Read the model definition and answer for the solid it produces. Units are mm, in the model's axes. A direction names the side the tool comes from. Give positions to 0.01 mm unless a question says otherwise; leave off trailing zeros. Loops run counter-clockwise (first coordinate to the right, second up) from the corner with the lowest first, then second, coordinate; pieces in that order, holes last. Notation, with made-up numbers: (-32.5, -16) - (-28.5, -16) arc R23 ccw to (-28.5, 0) - close; hole circle Ø10 at (-9.5, 42). An arc over 180 degrees is marked (long way). Use a Markdown table: item, result. Add a question column.
Item 1: A cutting plane is placed at B-B (y = -6.5). Determine the outline of the cut face in (x, z).
Item 2: For a pull along Z with two mould halves and no side action, classify faces 4 (the face through (24.2, 0.1, 0)), 5 (the face through (4.5, 25, 22.2)), 6 (the face through (-9.52, 23.52, 21.88)) as +Z half, -Z half, draft (parallel to the pull), parting line (faces both ways), or undercut.
Item 3: Each of these flat-tipped pins is pushed along its axis until it touches: P1, Ø0.6, axis at y = -24, z = 29.5, coming from the +X side; P2, Ø0.6, axis at y = 23, z = 1, coming from the +X side; P3, Ø3, axis at x = -17.33, z = 14, coming from the +Y side. Where does it stop, or does it pass through?
Item 4: Consider probe 1 along X at (y, z) = (12.5, 23.5); probe 2 along Y at (x, z) = (14, 24); probe 3 along X at (y, z) = (22.7, 14). Determine where each line is inside the solid, lowest interval first. Write a range as [from, to].
Item 5: Which of the six approach directions +Z, -Z, +X, -X, +Y, -Y give full straight-line access (tool end or side, diameter ignored) to faces 1 (the face through (-2, 24, 1)), 2 (the face through (-17.085, 22.799, 12.118)), 3 (the face through (-0.3, -22, 22.2))?
Item 6: A cutting plane is placed at A-A (x = 0). Determine the outline of the cut face in (y, z).
Item 7: A cutting plane is placed at D-D (z = 14). Give the number of separate pieces and of enclosed holes in the cut face, plus the area to 3 significant figures.
Item 8: A cutting plane is placed at C-C (z = 9.5). Determine the outline of the cut face in (x, y), plus the area to 3 significant figures.
from build123d import *

# Parameters (mm, degrees)
SKETCH1_W                                         = 53
SKETCH1_H                                         = 50
BOSS_EXTRUDE1_DEPTH                               = 28
FILLET1_R                                         = 5
SKETCH2_W                                         = 48
SKETCH2_H                                         = 44
CUT_EXTRUDE1_DEPTH                                = 28
SKETCH3_W                                         = 43
SKETCH3_H                                         = 3
BOSS_EXTRUDE2_DEPTH                               = 3
CUT_EXTRUDE2_DEPTH                                = 3
SKETCH10_R                                        = 8
CUT_EXTRUDE3_DEPTH                                = 3
CUT_EXTRUDE4_DEPTH                                = 3
CUT_EXTRUDE5_DEPTH                                = 3
MIRROR2_COPY_1_DEPTH                              = 3
SKETCH13_R                                        = 9
CUT_EXTRUDE12_DEPTH                               = 3
SKETCH14_R                                        = 3
CUT_EXTRUDE13_DEPTH                               = 3
SKETCH15_R                                        = 3
CUT_EXTRUDE14_DEPTH                               = 3
SKETCH39_W                                        = 4
SKETCH39_H                                        = 1
CUT_EXTRUDE15_DEPTH                               = 5
CSK_FOR_6_FLAT_HEAD_MACHINE_SCREW_100_D           = 3.7973
CSK_FOR_6_FLAT_HEAD_MACHINE_SCREW_100_DEPTH       = 3
CSK_FOR_6_FLAT_HEAD_MACHINE_SCREW_100_CSINK_D     = 7.0866
CSK_FOR_6_FLAT_HEAD_MACHINE_SCREW_100_CSINK_ANGLE = 100


with BuildPart() as part:
    # Sketch1 → Boss-Extrude1 (new body)
    with BuildSketch(Plane.XY):
        Rectangle(SKETCH1_W, SKETCH1_H)
    extrude(amount=BOSS_EXTRUDE1_DEPTH)

    # Fillet1
    fillet1_edges = [part.edges().sort_by_distance(p)[0] for p in [
        (26.5, -25, 14),
        (-26.5, -25, 14),
        (-26.5, 25, 14),
        (26.5, 25, 14),
    ]]
    fillet(fillet1_edges, radius=FILLET1_R)

    # Sketch2 → Cut-Extrude1 (cut)
    with BuildSketch(Plane.XY.offset(28)):
        Rectangle(SKETCH2_W, SKETCH2_H)
    extrude(amount=-CUT_EXTRUDE1_DEPTH, mode=Mode.SUBTRACT)

    # Sketch3 → Boss-Extrude2 (add)
    with BuildSketch(Plane.XY.offset(28)):
        with Locations((0, -23.5)):
            Rectangle(SKETCH3_W, SKETCH3_H)
    boss_extrude2 = extrude(amount=BOSS_EXTRUDE2_DEPTH)

    # Sketch9 → Cut-Extrude2 (cut)
    with BuildSketch(Plane.XZ.offset(25)):
        Polygon((21.5, 28), (18.5, 31), (21.5, 31), align=None)
    cut_extrude2 = extrude(amount=-CUT_EXTRUDE2_DEPTH, mode=Mode.SUBTRACT)

    # Mirror1: Cut-Extrude2 across plane
    add(cut_extrude2.mirror(Plane(origin=(0, 0, 0), x_dir=(0, 0, 1), z_dir=(1, 0, 0))), mode=Mode.SUBTRACT)

    # Sketch10 → Cut-Extrude3 (cut)
    with BuildSketch(Plane(origin=(0, -25, 0), x_dir=(-1, 0, 0), z_dir=(0, -1, 0))):
        with Locations(Location((0, -14, 0), (0, 0, 90))):
            Circle(SKETCH10_R)
    extrude(amount=-CUT_EXTRUDE3_DEPTH, mode=Mode.SUBTRACT)

    # Sketch11 → Cut-Extrude4 (cut)
    with BuildSketch(Plane.XZ.offset(25)):
        with BuildLine():
            Line((2, 31), (2, 29))
            ThreePointArc((2, 29), (0, 27), (-2, 29))
            Line((-2, 29), (-2, 31))
            ThreePointArc((-2, 31), (0, 33), (2, 31))
        make_face()
    cut_extrude4 = extrude(amount=-CUT_EXTRUDE4_DEPTH, mode=Mode.SUBTRACT)

    # Sketch12 → Cut-Extrude5 (cut)
    with BuildSketch(Plane.XZ.offset(25)):
        with BuildLine():
            Line((-2, 0), (-2, 2))
            ThreePointArc((-2, 2), (0, 4), (2, 2))
            Line((2, 2), (2, 0))
            ThreePointArc((2, 0), (0, -2), (-2, 0))
        make_face()
    cut_extrude5 = extrude(amount=-CUT_EXTRUDE5_DEPTH, mode=Mode.SUBTRACT)

    # Mirror2: Boss-Extrude2, Cut-Extrude2, Cut-Extrude4, Cut-Extrude5 across plane
    add(boss_extrude2.mirror(Plane.ZX))
    add(cut_extrude2.mirror(Plane.ZX), mode=Mode.SUBTRACT)
    add(cut_extrude4.mirror(Plane.ZX), mode=Mode.SUBTRACT)
    add(cut_extrude5.mirror(Plane.ZX), mode=Mode.SUBTRACT)

    # Mirror2 copy 1 sketch → Mirror2 copy 1 (cut)
    with BuildSketch(Plane(origin=(0, 25, 0), x_dir=(-1, 0, 0), z_dir=(0, 1, 0))):
        Polygon((21.5, 28), (18.5, 31), (21.5, 31), align=None)
    extrude(amount=-MIRROR2_COPY_1_DEPTH, mode=Mode.SUBTRACT)

    # Sketch13 → Cut-Extrude12 (cut)
    with BuildSketch(Plane(origin=(0, 25, 0), x_dir=(1, 0, 0), z_dir=(0, 1, 0))):
        with Locations(Location((0, -14, 0), (0, 0, 270))):
            Circle(SKETCH13_R)
    extrude(amount=-CUT_EXTRUDE12_DEPTH, mode=Mode.SUBTRACT)

    # Sketch14 → Cut-Extrude13 (cut)
    with BuildSketch(Plane(origin=(0, 25, 0), x_dir=(1, 0, 0), z_dir=(0, 1, 0))):
        with Locations(Location((-12.052516567, -20.270787808, 0), (0, 0, 270))):
            Circle(SKETCH14_R)
    cut_extrude13 = extrude(amount=-CUT_EXTRUDE13_DEPTH, mode=Mode.SUBTRACT)

    # Sketch15 → Cut-Extrude14 (cut)
    with BuildSketch(Plane(origin=(0, 25, 0), x_dir=(1, 0, 0), z_dir=(0, 1, 0))):
        with Locations(Location((-12.043222485, -7.723673845, 0), (0, 0, 270))):
            Circle(SKETCH15_R)
    cut_extrude14 = extrude(amount=-CUT_EXTRUDE14_DEPTH, mode=Mode.SUBTRACT)

    # Sketch39 → Cut-Extrude15 (cut)
    with BuildSketch(Plane(origin=(-24.285533906, 24.285533906, 0), x_dir=(0, 0, -1), z_dir=(-0.7071067811865464, 0.7071067811865488, 0))):
        with Locations((-13.86492965, 0)):
            Rectangle(SKETCH39_W, SKETCH39_H)
    cut_extrude15 = extrude(amount=-CUT_EXTRUDE15_DEPTH, mode=Mode.SUBTRACT)

    # CSK for #6 Flat Head Machine Screw (100)1
    with Locations(Plane(origin=(0, 25, 0), x_dir=(1, 0, 0), z_dir=(0, 1, 0))):
        with Locations((-17.332413571, -14)):
            csk_for_6_flat_head_machine_screw_100 = CounterSinkHole(CSK_FOR_6_FLAT_HEAD_MACHINE_SCREW_100_D / 2, CSK_FOR_6_FLAT_HEAD_MACHINE_SCREW_100_CSINK_D / 2, depth=CSK_FOR_6_FLAT_HEAD_MACHINE_SCREW_100_DEPTH, counter_sink_angle=CSK_FOR_6_FLAT_HEAD_MACHINE_SCREW_100_CSINK_ANGLE)

    # Mirror3: Cut-Extrude13, Cut-Extrude14, Cut-Extrude15, CSK for #6 Flat Head Machine Screw (100)1 across plane
    add(cut_extrude13.mirror(Plane(origin=(0, 0, 0), x_dir=(0, 0, 1), z_dir=(1, 0, 0))), mode=Mode.SUBTRACT)
    add(cut_extrude14.mirror(Plane(origin=(0, 0, 0), x_dir=(0, 0, 1), z_dir=(1, 0, 0))), mode=Mode.SUBTRACT)
    add(cut_extrude15.mirror(Plane(origin=(0, 0, 0), x_dir=(0, 0, 1), z_dir=(1, 0, 0))), mode=Mode.SUBTRACT)
    add(csk_for_6_flat_head_machine_screw_100.mirror(Plane(origin=(0, 0, 0), x_dir=(0, 0, 1), z_dir=(1, 0, 0))), mode=Mode.SUBTRACT)


solid = part.part
Geometry says:
| question | item | result |
|---|---|---|
| 1 | outline | (-26.5, 0) - (-24, 0) - (-24, 28) - (-26.5, 28) - close; (24, 0) - (26.5, 0) - (26.5, 28) - (24, 28) - close |
| 2 | face 4 | -Z half |
| 2 | face 5 | draft |
| 2 | face 6 | undercut |
| 3 | P1 | x = 20.3 |
| 3 | P2 | x = 25.71 |
| 3 | P3 | y = -22 |
| 4 | probe 1 | [-26.5, -24], [24, 26.5] |
| 4 | probe 2 | [-25, -22], [22, 25] |
| 4 | probe 3 | [-25.71, -23.41], [-21.99, -19.23], [-15.43, -9], [9, 15.43], [19.23, 21.99], [23.41, 25.71] |
| 5 | face 1 | -Z, +Y, -Y |
| 5 | face 2 | +Y |
| 5 | face 3 | +Z, -Z |
| 6 | outline | (-25, 4) - (-22, 4) - (-22, 6) - (-25, 6) - close; (-25, 22) - (-22, 22) - (-22, 27) - (-25, 27) - close; (22, 4) - (25, 4) - (25, 5) - (22, 5) - close; (22, 23) - (25, 23) - (25, 27) - (22, 27) - close |
| 7 | separate pieces | 6 |
| 7 | enclosed holes | 0 |
| 7 | area | 381 mm² |
| 8 | outline | (-26.5, -20) arc R5 ccw to (-21.5, -25) - (-6.61, -25) - (-6.61, -22) - (-24, -22) - (-24, 22) - (-14.46, 22) - (-14.46, 25) - (-21.5, 25) arc R5 ccw to (-26.5, 20) - close; (-9.63, 22) - (-7.79, 22) - (-7.79, 25) - (-9.63, 25) - close; (6.61, -25) - (21.5, -25) arc R5 ccw to (26.5, -20) - (26.5, 20) arc R5 ccw to (21.5, 25) - (14.46, 25) - (14.46, 22) - (24, 22) - (24, -22) - (6.61, -22) - close; (7.79, 22) - (9.63, 22) - (9.63, 25) - (7.79, 25) - close |
| 8 | area | 401 mm² |
